Model file for the job. Use its own axes, mm. Give positions to 0.01 mm unless a question says otherwise; leave off trailing zeros. Order: outer loops, then holes, each group sorted by start corner. A loop starts at its lowest first (then second) coordinate and runs counter-clockwise, first axis right, second up. Notation, with made-up numbers: M -24,57 L 29,57 A15 ccw 29,80 Z; hole C -17.5,-23 d10. An arc over 180 degrees is marked long. Return JSON: item names as keys, results as strings. Group by question number.
1. Wall check: probe 1 along Y at (x, z) = (98, 26); probe 2 along Y at (x, z) = (40, 17). Give the ranges that are in metal, low to high. Write a range as [from, to].
2. Slice it at B-B on z = 1. List the corners of the cut face in (x, y).
3. Slice it at A-A on z = 31. List the corners of the cut face in (x, y), then the cut area to 3 significant figures.
4. Pin check, flat tips, straight feed: pin 1 (8 mm diameter, centred on x = 215, z = 64, fed in from -Y); pin 2 (6 mm diameter, centred on y = 7, z = -0.5, fed in from +X); pin 3 (1 mm diameter, centred on x = 243, z = 8, fed in from -Y); pin 4 (5 mm diameter, centred on x = -108, y = 7, fed in from +Z). Stop position of each tip, or through.
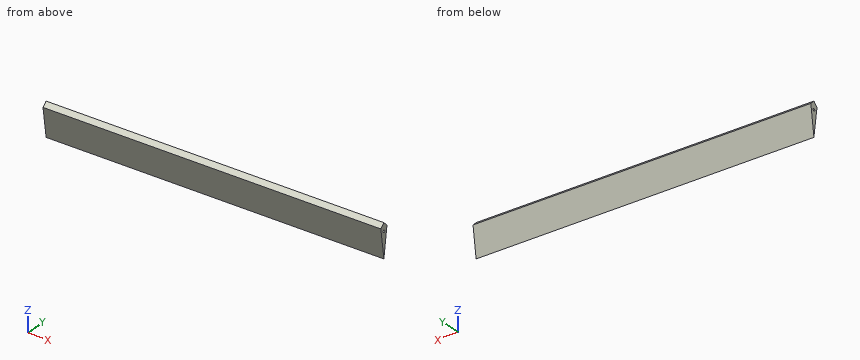
from build123d import *

# Parameters (mm, degrees)
AILERON_DEPTH           = 402.822020631
SKETCH2_R               = 2.75
CUT_EXTRUDE2_DEPTH      = 403.822020631
CUT_EXTRUDE2_DEPTH_BACK = 406.280098


with BuildPart() as part:
    # aileron_root → aileron (new body, symmetric, along a direction that is not the sketch's normal)
    with BuildSketch(Plane(origin=(0, 0, 0), x_dir=(0, 0, -1), z_dir=(1, 0, 0))):
        Polygon((-80, -10.846932253), (-80, 10.846932253), (0, 0), align=None)
    extrude(amount=AILERON_DEPTH, dir=(0.999527846, 0, 0.030725967), both=True)

    # Sketch2 → Cut-Extrude2 (cut, two sides)
    with BuildSketch(Plane(origin=(0, 0, 0), x_dir=(-0.030725967, 0, 0.999527846), z_dir=(-0.999527846, 0, -0.030725967))) as cut_extrude2_sk:
        with Locations((60, 0)):
            Circle(SKETCH2_R)
        Polygon((78.962227681, 0), (68.115295428, -10.846932253), (79.962227681, -10.846932253), (79.962227681, 10.846932253), (68.115295428, 10.846932253), align=None)
    extrude(amount=CUT_EXTRUDE2_DEPTH, mode=Mode.SUBTRACT)
    extrude(cut_extrude2_sk.sketch, amount=-CUT_EXTRUDE2_DEPTH_BACK, mode=Mode.SUBTRACT)


solid = part.part
Result:
{
 "1": {"probe 1": "y = [-3.12, 3.12]", "probe 2": "y = [-2.14, 2.14]"},
 "2": {"outline": "M -402.63,-1.81 L 32.53,0 L -402.63,1.81 Z"},
 "3": {"outline": "M -402.63,-5.88 L 402.63,-2.53 L 402.63,2.53 L -402.63,5.88 Z", "area": "6,770 mm2"},
 "4": {"pin 1": "stops at y = -8.32", "pin 2": "passes through", "pin 3": "stops at y = -0.14", "pin 4": "stops at z = 71.18"}
}
